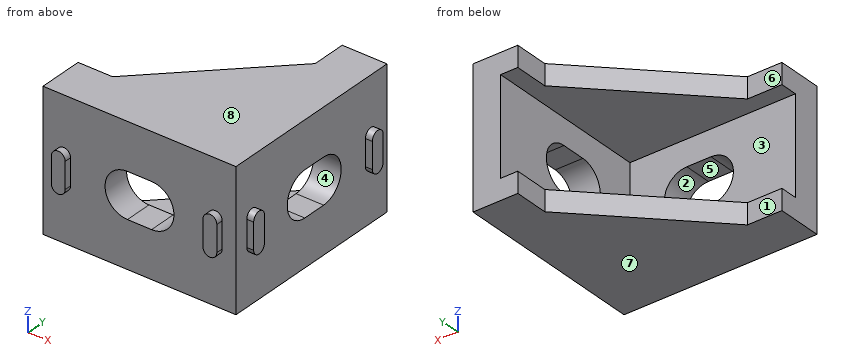
Autodesk Inventor part; units mm, degrees
ref_plane "YZ Plane" through (0, 0, 0) normal (1, 0, 0) x (0, 1, 0)
ref_plane "XZ Plane" through (0, 0, 0) normal (0, 1, 0) x (-1, 0, 0)
ref_plane "XY Plane" through (0, 0, 0) normal (0, 0, 1) x (1, 0, 0)
sketch "Sketch1" plane through (0, 0, 0) normal (0, 1, 0) x (-1, 0, 0)
  line L0 (0, 0) -> (28, 0)
  line L1 (28, 0) -> (28, -20)
  line L2 (28, -20) -> (0, -20)
  line L3 (0, -20) -> (0, 0)
  dimension "d0" = 28
  dimension "d1" = 20
extrude "Extrusion1" add sketch "Sketch1" along normal blind 4
sketch "Sketch2" plane through (0, 4, 0) normal (0, 1, 0) x (1, 0, 0)
  line L0 (0, 20) -> (-28, 20)
  line L1 (-28, 20) -> (-28, 0)
  line L2 (-28, 0) -> (0, 0)
  line L3 (0, 0) -> (0, 20)
  line L4 (0, 0) -> (-4, 0)
  line L5 (-4, 0) -> (-4, 20)
  line L6 (-4, 20) -> (0, 20)
  line L7 (0, 20) -> (0, 0)
  dimension "d4" = 4
extrude "Extrusion2" add sketch "Sketch2" along normal blind 24 contours L3 L2 L5 L0
sketch "Sketch3" plane through (-4, 4, -20) normal (-1, 0, 0) x (0, 0, 1)
  line L0 (20, -4) -> (0, -4)
  line L1 (0, -4) -> (0, 24)
  line L2 (20, 24) -> (0, 24)
  line L3 (20, -4) -> (20, 24)
  line L4 (0, -4) -> (0, 24)
  line L5 (10, 15.5) -> (10, 15.5)
  line L6 (13.25, 12.25) -> (13.25, 8.75)
  line L7 (10, 5.5) -> (10, 5.5)
  line L8 (6.75, 8.75) -> (6.75, 12.25)
  line L9 (6.75, 15.5) -> (13.25, 5.5) construction
  line L10 (13.25, 15.5) -> (6.75, 5.5) construction
  arc A0 (10, 5.5) -> (13.25, 8.75) centre (10, 8.75) ccw
  arc A1 (6.75, 8.75) -> (10, 5.5) centre (10, 8.75) ccw
  arc A2 (13.25, 12.25) -> (10, 15.5) centre (10, 12.25) ccw
  arc A3 (10, 15.5) -> (6.75, 12.25) centre (10, 12.25) ccw
  point P0 (10, 10.5)
  point P1 (10, 15.5)
  dimension "d7" = 6.5
  dimension "d8" = 10
  dimension "d9" = 3.25
  dimension "d10" = 3.25
  dimension "d11" = 3.25
extrude "Extrusion3" cut sketch "Sketch3" against normal blind 4 contours L6 A0 A1 L8 A3 A2
sketch "Sketch4" plane through (0, 4, 0) normal (0, 1, 0) x (1, 0, 0)
  line L0 (0, 20) -> (-28, 20)
  line L1 (0, 0) -> (0, 20)
  line L2 (-28, 0) -> (0, 0)
  line L3 (-28, 20) -> (-28, 0)
  line L4 (-15.75, 6.75) -> (-12.25, 6.75)
  line L5 (-9, 10) -> (-9, 10)
  line L6 (-12.25, 13.25) -> (-15.75, 13.25)
  line L7 (-19, 10) -> (-19, 10)
  line L8 (-19, 6.75) -> (-9, 13.25) construction
  line L9 (-9, 6.75) -> (-19, 13.25) construction
  arc A0 (-9, 10) -> (-12.25, 13.25) centre (-12.25, 10) ccw
  arc A1 (-12.25, 6.75) -> (-9, 10) centre (-12.25, 10) ccw
  arc A2 (-15.75, 13.25) -> (-19, 10) centre (-15.75, 10) ccw
  arc A3 (-19, 10) -> (-15.75, 6.75) centre (-15.75, 10) ccw
  point P0 (-14, 10)
  dimension "d14" = 10
  dimension "d15" = 6.5
  dimension "d16" = 3.25
extrude "Extrusion4" cut sketch "Sketch4" against normal blind 4 contours A3 A2 L6 A0 A1 L4
sketch "Sketch5" plane through (0, 0, -20) normal (0, 0, -1) x (-1, 0, 0)
  line L0 (0, 0) -> (28, 0)
  line L1 (28, 0) -> (28, 4)
  line L2 (4, 4) -> (28, 4)
  line L3 (4, 4) -> (4, 28)
  line L4 (0, 28) -> (4, 28)
  line L5 (0, 0) -> (0, 28)
  line L6 (0, 28) -> (6.5, 28)
  line L7 (28, 0) -> (28, 6.5)
  line L8 (28, 6.5) -> (23, 6.5)
  line L9 (6.5, 28) -> (6.5, 23)
  line L10 (6.5, 23) -> (23, 6.5)
  dimension "d19" = 6.5
  dimension "d20" = 6.5
  dimension "d21" = 5
  dimension "d22" = 5
extrude "Extrusion5" add sketch "Sketch5" against normal blind 3 contours L2 L3 L6 L9 L10 L8 L7
sketch "Sketch6" plane through (-28, 0, 0) normal (0, 0, 1) x (1, 0, 0)
  line L0 (21.5, 23) -> (5, 6.5)
  line L1 (5, 6.5) -> (0, 6.5)
  line L2 (0, 6.5) -> (0, 4)
  line L3 (24, 4) -> (0, 4)
  line L4 (24, 28) -> (24, 4)
  line L5 (24, 28) -> (21.5, 28)
  line L6 (21.5, 28) -> (21.5, 23)
  line L7 (0, 0) -> (28, 0)
  line L8 (28, 0) -> (28, 28)
  line L9 (24, 28) -> (28, 28)
  line L10 (24, 4) -> (24, 28)
  line L11 (0, 4) -> (24, 4)
  line L12 (0, 0) -> (0, 4)
extrude "Extrusion6" add sketch "Sketch6" against normal blind 3 contours L6 L5 L4 L3 L2 L1 L0
sketch "Sketch7" plane through (0, 0, 0) normal (1, 0, 0) x (0, 0, -1)
  line L0 (3, 4) -> (17, 4)
  line L1 (10, 4) -> (10, 3)
  line L2 (8.1, 2) -> (11.9, 2)
  line L3 (12.9, 3) -> (12.9, 3)
  line L4 (11.9, 4) -> (8.1, 4)
  line L5 (7.1, 3) -> (7.1, 3)
  line L6 (7.1, 2) -> (12.9, 4) construction
  line L7 (12.9, 2) -> (7.1, 4) construction
  arc A0 (8.1, 4) -> (7.1, 3) centre (8.1, 3) ccw
  arc A1 (7.1, 3) -> (8.1, 2) centre (8.1, 3) ccw
  arc A2 (12.9, 3) -> (11.9, 4) centre (11.9, 3) ccw
  arc A3 (11.9, 2) -> (12.9, 3) centre (11.9, 3) ccw
  point P0 (0, 0)
  dimension "d27" = 1
  dimension "d28" = 5.8
  dimension "d29" = 1
extrude "Extrusion7" add sketch "Sketch7" along normal blind 1
sketch "Sketch8" plane through (0, 0, 0) normal (0, -1, 0) x (1, 0, 0)
  line L0 (-4, -3) -> (-4, -17)
  line L1 (-4, -10) -> (-3, -10)
  line L2 (-3, -7.1) -> (-3, -7.1)
  line L3 (-4, -8.1) -> (-4, -11.9)
  line L4 (-3, -12.9) -> (-3, -12.9)
  line L5 (-2, -11.9) -> (-2, -8.1)
  line L6 (-2, -7.1) -> (-4, -12.9) construction
  line L7 (-4, -7.1) -> (-2, -12.9) construction
  arc A0 (-4, -11.9) -> (-3, -12.9) centre (-3, -11.9) ccw
  arc A1 (-3, -12.9) -> (-2, -11.9) centre (-3, -11.9) ccw
  arc A2 (-2, -8.1) -> (-3, -7.1) centre (-3, -8.1) ccw
  arc A3 (-3, -7.1) -> (-4, -8.1) centre (-3, -8.1) ccw
  point P0 (0, 0)
  dimension "d32" = 1
  dimension "d33" = 5.8
  dimension "d34" = 1
extrude "Extrusion8" add sketch "Sketch8" along normal blind 1
sketch "Sketch9" plane through (0, 0, 0) normal (0, -1, 0) x (1, 0, 0)
  line L0 (-28, -20) -> (-28, 0)
  line L1 (-28, -10) -> (-25, -10)
  line L2 (-25, -12.9) -> (-25, -12.9)
  line L3 (-26, -11.9) -> (-26, -8.1)
  line L4 (-25, -7.1) -> (-25, -7.1)
  line L5 (-24, -8.1) -> (-24, -11.9)
  line L6 (-24, -12.9) -> (-26, -7.1) construction
  line L7 (-26, -12.9) -> (-24, -7.1) construction
  arc A0 (-26, -11.9) -> (-25, -12.9) centre (-25, -11.9) ccw
  arc A1 (-25, -7.1) -> (-26, -8.1) centre (-25, -8.1) ccw
  arc A2 (-24, -8.1) -> (-25, -7.1) centre (-25, -8.1) ccw
  arc A3 (-25, -12.9) -> (-24, -11.9) centre (-25, -11.9) ccw
  point P0 (0, 0)
  dimension "d37" = 3
  dimension "d38" = 2
  dimension "d39" = 5.8
  dimension "d40" = 1
extrude "Extrusion9" add sketch "Sketch9" along normal blind 1
sketch "Sketch10" plane through (0, 0, 0) normal (1, 0, 0) x (0, 0, -1)
  line L0 (17, 28) -> (3, 28)
  line L1 (10, 28) -> (10, 25)
  line L2 (8.1, 24) -> (11.9, 24)
  line L3 (12.9, 25) -> (12.9, 25)
  line L4 (11.9, 26) -> (8.1, 26)
  line L5 (7.1, 25) -> (7.1, 25)
  line L6 (7.1, 24) -> (12.9, 26) construction
  line L7 (12.9, 24) -> (7.1, 26) construction
  arc A0 (8.1, 26) -> (7.1, 25) centre (8.1, 25) ccw
  arc A1 (12.9, 25) -> (11.9, 26) centre (11.9, 25) ccw
  arc A2 (11.9, 24) -> (12.9, 25) centre (11.9, 25) ccw
  arc A3 (7.1, 25) -> (8.1, 24) centre (8.1, 25) ccw
  point P0 (0, 0)
  dimension "d43" = 3
  dimension "d44" = 5.8
  dimension "d45" = 2
  dimension "d46" = 1
extrude "Extrusion10" add sketch "Sketch10" along normal blind 1
properties part number "CORNER2028"
Input: part model. Units: mm. Frame: model coordinates. Face numbers are marked on the shaded views. A direction names the side the tool comes from. Coordinates: 2 decimals unless noted, no trailing zeros. Loops run counter-clockwise (first coordinate to the right, second up) from the corner with the lowest first, then second, coordinate; pieces in that order, holes last. Notation, with made-up numbers: M -25,35.25 L 33,35.25 A24 cw 33,59.25 Z; hole C 16.25,36.5 d4. An arc over 180 degrees is marked long. Answer in a Markdown table with one row per item.
1. Material intervals for line 1 (Z direction, x = -19, y = 10); line 2 (X direction, y = 21, z = -7.5); line 3 (Y direction, x = -19.75, z = -11), sorted ascending.
Response:
| item | result |
|---|---|
| line 1 | z = -20 to -17, -3 to 0 |
| line 2 | x = -4 to 0 |
| line 3 | y = 0 to 4 |
2. Section D-D, the plane x = -22.25. Output: boundary loops of the cut face in (y, z).
Response:
| item | result |
|---|---|
| outline | M 0,-20 L 7.25,-20 L 7.25,-17 L 4,-17 L 4,-3 L 7.25,-3 L 7.25,0 L 0,0 Z |
3. Draft query along Z for the marked faces 5, 6, 7 and 8. Return one class per face: pulls with the +Z half, pulls with the -Z half, needs draft (parallel to the pull), parting line crosses it, or undercut.
Response:
| item | result |
|---|---|
| face 5 | undercut |
| face 6 | needs draft |
| face 7 | pulls with the -Z half |
| face 8 | pulls with the +Z half |
4. Section A-A, the plane y = 3. Output: boundary loops of the cut face in (x, z).
Response:
| item | result |
|---|---|
| outline | M -28,-20 L 0,-20 L 0,-12.9 L 1,-12.9 L 1,-7.1 L 0,-7.1 L 0,0 L -28,0 Z; hole M -15.75,-13.25 L -12.25,-13.25 A3.25 ccw -12.25,-6.75 L -15.75,-6.75 A3.25 ccw Z |
5. First-contact query: pin 1 (0.5 mm diameter, centred on y = -0.5, z = -10.5, fed in from -X); pin 2 (6 mm diameter, centred on y = 15.5, z = -8.5, fed in from +X); pin 3 (10 mm diameter, centred on x = -15.5, z = -13.5, fed in from -Y). Flat tips, straight axial feed; report the tip coordinate or a pass-through.
Response:
| item | result |
|---|---|
| pin 1 | stops at x = -26 |
| pin 2 | stops at x = 0 |
| pin 3 | stops at y = 0 |
6. Section C-C, the plane z = -10. Count the separate pieces of the cut face and the enclosed holes in it, then the cut area to 3 significant figures.
Response:
| item | result |
|---|---|
| separate pieces | 3 |
| enclosed holes | 0 |
| area | 136 mm2 |
7. Reachability of the marked faces 1, 2, 3 and 4 from +Z, -Z, +X, -X, +Y, -Y: full face, straight path, thin tool, end or side. Return the list, or none.
Response:
| item | result |
|---|---|
| face 1 | +Z, -Z, -X, +Y |
| face 2 | +Y, -Y |
| face 3 | -X, +Y |
| face 4 | +X, -X |
8. Section B-B, the plane x = -14. Output: boundary loops of the cut face in (y, z).
Response:
| item | result |
|---|---|
| outline | M 0,-20 L 15.5,-20 L 15.5,-17 L 4,-17 L 4,-13.25 L 0,-13.25 Z; M 0,-6.75 L 4,-6.75 L 4,-3 L 15.5,-3 L 15.5,0 L 0,0 Z |
